Can you work these out from the model? Positions are in its coordinate system, mm. Round coordinates to 2 decimals unless told otherwise and drop trailing zeros. Order: outer loops, then holes, each group sorted by start corner. A loop starts at its lowest first (then second) coordinate and runs counter-clockwise, first axis right, second up. Notation, with made-up numbers: (52, -9.5) -> (104, -9.5) arc R26 ccw to (104, 28.5) -> close; hole circle Ø2 at (45.25, -10.5). An arc over 180 degrees is marked (long way). Use a Markdown table: item, result. Add a question column.
Q1. If we section it at A-A on x = 14: List the corners of the cut face in (y, z) for me.
Q2. I need wall thicknesses on line 1 along X through (y, z) = (41, 2.25); line 2 along X through (y, z) = (44, 0.4); line 3 along Y through (x, z) = (12, 1.25). Which ranges of each line are inside material? Lowest first, please. Write a range as [from, to].
Q3. If we section it at B-B on y = 52.5: List the corners of the cut face in (x, z) for me, plus the area to 3 significant figures.
Q4. I'm going to push flat-ended pins straight in: pin 1 Ø0.9 at (y, z) = (43.5, 1) entering from +X; pin 2 Ø3 at (x, y) = (13.21, 57.76) entering from -Z; pin 3 Ø1.5 at (x, z) = (42, 2) entering from +Y. Where does each tip first touch, or does it pass through?
Q5. If we section it at D-D on x = 36: List the corners of the cut face in (y, z) for me.
Q6. If we section it at C-C on z = 2.2: List the corners of the cut face in (x, y) for me, plus the area to 3 significant figures.
```python
from build123d import *

# Parameters (mm, degrees)
F1_DEPTH = 3
F2_R     = 2.5
F3_DEPTH = 25.4


with BuildPart() as f1:
    # F0 (on Top) → F1 (new body)
    with BuildSketch(Plane.XY):
        Polygon((39.395284, 37.122335), (39.473195, 27.290761), (57.550997, 27.290761), (57.550997, 36.883935), (53.969547, 36.883935), (53.969547, 51.678739), (57.550997, 51.678739), (57.550997, 61.335869), (43.289147, 61.335869), (33.674654, 47.990695), (23.932254, 61.335869), (9.627766, 61.335869), (9.627766, 51.678739), (13.251853, 51.678739), (13.251853, 36.883935), (9.627766, 36.883935), (9.627766, 27.290761), (27.743142, 27.290761), (27.743142, 36.883935), (23.932254, 36.883935), (23.932254, 46.157219), (33.468755, 33.094085), (43.289147, 46.282709), (43.289147, 37.122335), align=None)
    extrude(amount=F1_DEPTH)

    # F2 (on face) → F3 (cut)
    with BuildSketch(Plane.XY.offset(3)):
        with Locations((13.209973, 57.75835)):
            Circle(F2_R)
    extrude(amount=-F3_DEPTH, mode=Mode.SUBTRACT)


solid = f1.part
```
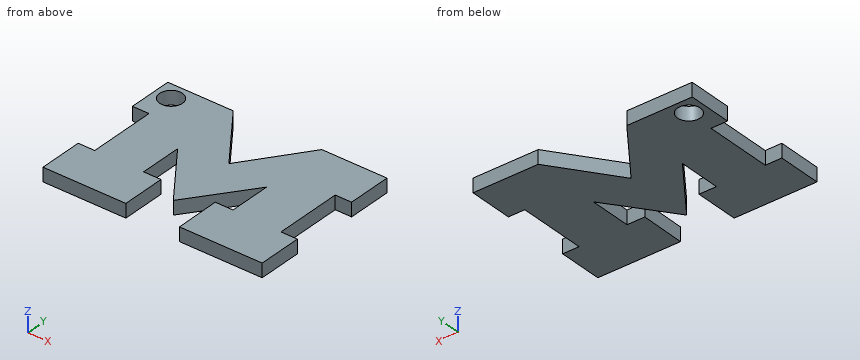
Answer below:
| question | item | result |
|---|---|---|
| 1 | outline | (27.29, 0) -> (55.39, 0) -> (55.39, 3) -> (27.29, 3) -> close; (60.13, 0) -> (61.34, 0) -> (61.34, 3) -> (60.13, 3) -> close |
| 2 | line 1 | [13.25, 23.93], [27.7, 39.36], [43.29, 53.97] |
| 2 | line 2 | [13.25, 23.93], [25.51, 41.59], [43.29, 53.97] |
| 2 | line 3 | [27.29, 36.88], [51.68, 55.57], [59.95, 61.34] |
| 3 | outline | (9.63, 0) -> (30.38, 0) -> (30.38, 3) -> (9.63, 3) -> close; (36.92, 0) -> (57.55, 0) -> (57.55, 3) -> (36.92, 3) -> close |
| 3 | area | 124 mm² |
| 4 | pin 1 | x = 53.97 |
| 4 | pin 2 | through |
| 4 | pin 3 | y = 60.59 |
| 5 | outline | (36.49, 0) -> (51.22, 0) -> (51.22, 3) -> (36.49, 3) -> close |
| 6 | outline | (9.63, 27.29) -> (27.74, 27.29) -> (27.74, 36.88) -> (23.93, 36.88) -> (23.93, 46.16) -> (33.47, 33.09) -> (43.29, 46.28) -> (43.29, 37.12) -> (39.4, 37.12) -> (39.47, 27.29) -> (57.55, 27.29) -> (57.55, 36.88) -> (53.97, 36.88) -> (53.97, 51.68) -> (57.55, 51.68) -> (57.55, 61.34) -> (43.29, 61.34) -> (33.67, 47.99) -> (23.93, 61.34) -> (9.63, 61.34) -> (9.63, 51.68) -> (13.25, 51.68) -> (13.25, 36.88) -> (9.63, 36.88) -> close; hole circle Ø5 at (13.21, 57.76) |
| 6 | area | 1,210 mm² |
